```python
from build123d import *

# Parameters (mm, degrees)
SKETCH1_W           = 5
SKETCH1_H           = 5
BOSS_EXTRUDE1_DEPTH = 8
SKETCH2_W           = 2
SKETCH2_H           = 3
CUT_EXTRUDE1_DEPTH  = 1
SKETCH4_W           = 1
SKETCH4_H           = 4
CUT_EXTRUDE4_DEPTH  = 4
SKETCH5_W           = 1
SKETCH5_H           = 2
CUT_EXTRUDE5_DEPTH  = 3
CUT_EXTRUDE6_DEPTH  = 3
SKETCH7_W           = 2
SKETCH7_H           = 1
CUT_EXTRUDE7_DEPTH  = 1
CUT_EXTRUDE8_DEPTH  = 2
CUT_EXTRUDE9_DEPTH  = 2
CUT_EXTRUDE10_DEPTH = 2


with BuildPart() as part:
    # Sketch1 → Boss-Extrude1 (new body)
    with BuildSketch(Plane.XY):
        Rectangle(SKETCH1_W, SKETCH1_H)
    extrude(amount=BOSS_EXTRUDE1_DEPTH)

    # Sketch2 → Cut-Extrude1 (cut)
    with BuildSketch(Plane(origin=(0, 2.5, 0), x_dir=(1, 0, 0), z_dir=(0, 1, 0))):
        with Locations((-1.5, -4.5)):
            Rectangle(SKETCH2_W, SKETCH2_H)
    extrude(amount=-CUT_EXTRUDE1_DEPTH, mode=Mode.SUBTRACT)

    # Sketch4 → Cut-Extrude4 (cut)
    with BuildSketch(Plane(origin=(2.5, 0, 0), x_dir=(0, 0, -1), z_dir=(1, 0, 0))):
        with Locations((-7.5, -0.5)):
            Rectangle(SKETCH4_W, SKETCH4_H)
    extrude(amount=-CUT_EXTRUDE4_DEPTH, mode=Mode.SUBTRACT)

    # Sketch5 → Cut-Extrude5 (cut)
    with BuildSketch(Plane(origin=(2.5, 0, 0), x_dir=(0, 0, -1), z_dir=(1, 0, 0))):
        with Locations((-6.5, -1.5)):
            Rectangle(SKETCH5_W, SKETCH5_H)
    extrude(amount=-CUT_EXTRUDE5_DEPTH, mode=Mode.SUBTRACT)

    # Sketch6 → Cut-Extrude6 (cut)
    with BuildSketch(Plane(origin=(2.5, 0, 0), x_dir=(0, 0, -1), z_dir=(1, 0, 0))):
        Polygon((-8, 1.5), (-8, 2.5), (-1, 2.5), (-1, 0.5), (-3, 0.5), (-3, -0.5), (-6, -0.5), (-7, -0.5), (-7, 1.5), align=None)
    extrude(amount=-CUT_EXTRUDE6_DEPTH, mode=Mode.SUBTRACT)

    # Sketch7 → Cut-Extrude7 (cut)
    with BuildSketch(Plane.XY.offset(6)):
        with Locations((1.5, -1)):
            Rectangle(SKETCH7_W, SKETCH7_H)
    extrude(amount=-CUT_EXTRUDE7_DEPTH, mode=Mode.SUBTRACT)

    # Sketch8 → Cut-Extrude8 (cut)
    with BuildSketch(Plane(origin=(0, 0, 0), x_dir=(-1, 0, 0), z_dir=(0, 0, -1))):
        Polygon((-0.5, 2.5), (-1.5, 1.5), (-1.5, -2.5), (-2.5, -2.5), (-2.5, 2.5), align=None)
    extrude(amount=-CUT_EXTRUDE8_DEPTH, mode=Mode.SUBTRACT)

    # Sketch9 → Cut-Extrude9 (cut)
    with BuildSketch(Plane.XY.offset(3)):
        Polygon((0.5, 0.5), (1.5, -0.5), (2.5, -0.5), (2.5, 0.5), align=None)
    extrude(amount=-CUT_EXTRUDE9_DEPTH, mode=Mode.SUBTRACT)

    # Sketch10 → Cut-Extrude10 (cut)
    with BuildSketch(Plane(origin=(0, 0, 2), x_dir=(-1, 0, 0), z_dir=(0, 0, -1))):
        Polygon((-1.5, -0.5), (-2.5, -1.5), (-2.5, -0.5), align=None)
    extrude(amount=-CUT_EXTRUDE10_DEPTH, mode=Mode.SUBTRACT)


solid = part.part
```
Check sheet for the modelled part. Datum: model origin and axes. Units: mm. A direction names the side the tool comes from. Coordinates: 2 decimals unless noted, no trailing zeros. Loops run counter-clockwise (first coordinate to the right, second up) from the corner with the lowest first, then second, coordinate; pieces in that order, holes last. Notation, with made-up numbers: M 23,-9.5 L 81,-9.5 A11 cw 81,-3.5 Z; hole C 33,40 d1. An arc over 180 degrees is marked long. Answer as a JSON object with one key per item and string values.
1. Sectioned sample at D-D on z = 5.25. Record the cut outline in (x, y), and give its area (3 significant figures).
Outcome:
{"outline": "M -2.5,-2.5 L 2.5,-2.5 L 2.5,-1.5 L 0.5,-1.5 L 0.5,-0.5 L -0.5,-0.5 L -0.5,1.5 L -2.5,1.5 Z", "area": "12.0 mm²"}
2. Sectioned sample at C-C on y = -0.25. Record the cut outline in (x, z), and give its area (3 significant figures).
Outcome:
{"outline": "M -2.5,0 L 1.5,0 L 1.5,1 L 1.25,1 L 1.25,3 L -0.5,3 L -0.5,7 L -1.5,7 L -1.5,8 L -2.5,8 Z", "area": "20.5 mm²"}
3. Scan lines: L1, parallel to Z at x = -1.7, y = 1.9; L2, parallel to Y at x = -1.8, z = 5.5; L3, parallel to Z at x = 0.15, y = -1.6. Record each from-to range of solid material in increasing order. Write a range as from..to.
Outcome:
{"L1": "0..3, 6..8", "L2": "-2.5..1.5", "L3": "0..6"}
4. Release check for a two-part mould opening along Z. For faces 5 (the flat face through (-2, 2, 6)), 6 (the flat face through (-1, 1.5, 7.5)), 7 (the flat face through (2.2, -0.8, 4)) record: pulls with the +Z half, pulls with the -Z half, needs draft (parallel to the pull), parting line crosses it, or undercut.
Outcome:
{"face 5": "undercut", "face 6": "needs draft", "face 7": "pulls with the -Z half"}
5. Access from +Z, -Z, +X, -X, +Y, -Y to the whole of each face (thin tool, end or side, straight path). Record for faces 1 (the flat face through (-1.5, -0.5, 7.5)), 2 (the flat face through (1.5, -1, 1)), 3 (the flat face through (1.5, -0.5, 2.5)), 4 (the flat face through (0, 0, 3)).
Outcome:
{"face 1": "+Z, +X, -Y", "face 2": "-Z, +X, +Y, -Y", "face 3": "+X, +Y", "face 4": "+Z, +X, +Y"}
6. Sectioned sample at B-B on x = -0.85. Record the cut outline in (y, z), and give its area (3 significant figures).
Outcome:
{"outline": "M -2.5,0 L 2.5,0 L 2.5,3 L 1.5,3 L 1.5,6 L 2.5,6 L 2.5,8 L 1.5,8 L 1.5,7 L -2.5,7 Z", "area": "33.0 mm²"}
7. Depth check by flat-ended pin: P1, Ø1.1, axis at x = -2, y = 2, coming from the -Z side; P2, Ø2.5, axis at x = 0.5, z = 5, coming from the +Y side; P3, Ø0.8, axis at x = 1, y = 0, coming from the +Z side; P4, Ø0.8, axis at x = 2, y = -1, coming from the +Z side. Enter the tip coordinate at first touch or a pass-through.
Outcome:
{"P1": "z = 0", "P2": "y = 1.5", "P3": "z = 3", "P4": "z = 5"}
8. Sectioned sample at A-A on y = 2. Record the cut outline in (x, z), and give its area (3 significant figures).
Outcome:
{"outline": "M -2.5,0 L 1,0 L 1,1 L -0.5,1 L -0.5,3 L -2.5,3 Z; M -2.5,6 L -0.5,6 L -0.5,8 L -2.5,8 Z", "area": "11.5 mm²"}
